The listing builds one solid part. Answer for the finished solid, in the listing's coordinates (mm). Coordinates: 2 decimals unless noted, no trailing zeros. Write each loop counter-clockwise with the first axis right and the second up, starting at its lowest first coordinate (ties: lowest second). Pieces come first, ordered by that corner, then holes.
from build123d import *

# Parameters (mm, degrees)
BOSS_EXTRUDE2_DEPTH = 24
FILLET3_R           = 2


with BuildPart() as part:
    # Sketch2 → Boss-Extrude2 (new body)
    with BuildSketch(Plane(origin=(0, 0, 0), x_dir=(1, 0, 0), z_dir=(0, 1, 0))):
        with BuildLine():
            ThreePointArc((64.008898715, 11.143267641), (64.514374858, 13.892879926), (63.719057289, 16.573056006))
            ThreePointArc((63.719057289, 16.573056006), (60.499660734, 16.149214409), (58.522904866, 13.573056006))
            ThreePointArc((58.522904866, 13.573056006), (43.615754555, -4.011786119), (21.55946325, -10.71773995))
            ThreePointArc((21.55946325, -10.71773995), (18.586355818, -13.744393581), (21.613009449, -16.717501013))
            ThreePointArc((21.613009449, -16.717501013), (46.910872497, -9.025985731), (64.008898715, 11.143267641))
        make_face()
    extrude(amount=BOSS_EXTRUDE2_DEPTH)

    # Fillet3
    fillet3_edges = [part.edges().sort_by_distance(p)[0] for p in [
        (63.719057289, 12, -16.573056006),
    ]]
    fillet(fillet3_edges, radius=FILLET3_R)


solid = part.part
Q1. The part is cut by section B-B, the plane x = 30. Write down the section's boundary in (y, z).
Answers below:
outline: (0, 9.76) - (24, 9.76) - (24, 15.88) - (0, 15.88) - close
Q2. Find the intervals of material crossed by probe 1 along Z at (x, y) = (45, 10.25); probe 2 along Z at (x, y) = (28, 15); probe 3 along X at (y, z) = (9, -5.5), in increasing order.
Answers below:
probe 1: z = 3.06 to 10.22
probe 2: z = 10.15 to 16.22
probe 3: x = 53.77 to 61.03
Q3. The part is cut by section A-A, the plane z = -7. Write down the section's boundary in (x, y).
Answers below:
outline: (54.85, 0) - (61.92, 0) - (61.92, 24) - (54.85, 24) - close
Q4. Given pin 1 (3 mm diameter, centred on y = 2.5, z = -4.5, fed in from -X); pin 2 (3 mm diameter, centred on y = 7, z = -3.5, fed in from -X); pin 3 (1.5 mm diameter, centred on x = 36, y = 7.5, fed in from +Z), each flat-ended and moving along its own axis, determine where each tip first touches the part or whether it passes through.
Answers below:
pin 1: stops at x = 51.72
pin 2: stops at x = 50.81
pin 3: stops at z = 14.56
